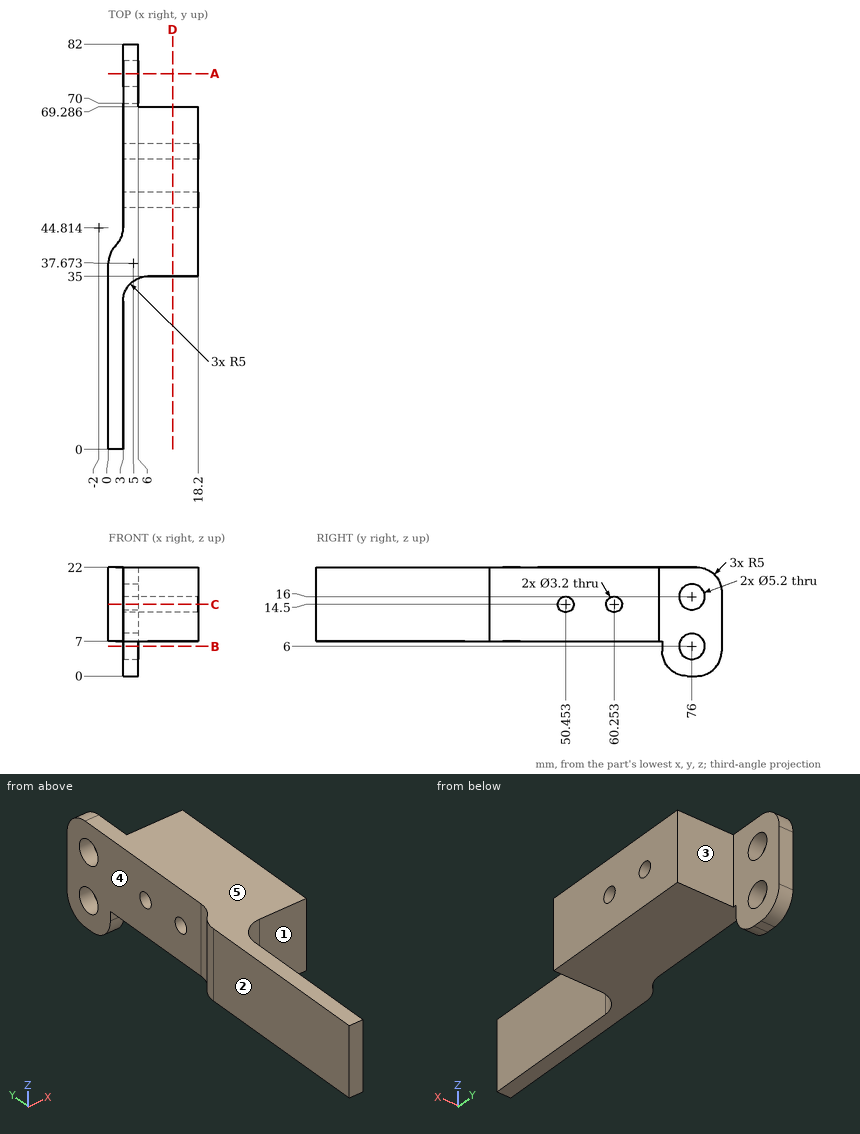
The drawing under review shows one solid part. Ordinate dimensions are in mm from its lowest x, y, z. A direction names the side the tool comes from. Give positions to 0.01 mm unless a question says otherwise; leave off trailing zeros. Loops run counter-clockwise (first coordinate to the right, second up) from the corner with the lowest first, then second, coordinate; pieces in that order, holes last. Notation, with made-up numbers: M 58,12.5 L 73,12.5 A35 cw 73,45.5 Z; hole C 55.25,-31.75 d1. An arc over 180 degrees is marked long. Return JSON: item names as keys, results as strings. Group by question number.
Item 1: We need section C-C (z = 14.5). Give the boundary of the cut face in (x, y).
Item 2: We need section A-A (y = 76). Give the boundary of the cut face in (x, z), and give its area (3 significant figures).
Item 3: We need section B-B (z = 6). Give the boundary of the cut face in (x, y), and give its area (3 significant figures).
Item 4: For probe 1 along Z at (x, y) = (13, 50.5); probe 2 along Y at (x, z) = (3.65, 6); probe 3 along Y at (x, z) = (11.75, 21.25), list the stretches that pass through material, from the lowest coordinate up.
Item 5: Insertion check: pin 1 Ø12 at (y, z) = (17, 11.5) entering from +X; pin 2 Ø6.5 at (y, z) = (77.5, 8) entering from +X; pin 3 Ø1.6 at (x, z) = (4.5, 6) entering from -Y. Each pin has a flat end and moves straight along its axis. Give the tip position at first contact, or say it passes through.
Item 6: Tool access review of the marked faces 1, 2, 3, 4 and 5: name each direction out of +Z, -Z, +X, -X, +Y, -Y from which nothing blocks a thin tool from reaching the whole face with its end or side.
Item 7: We need section D-D (x = 13). Give the boundary of the cut face in (y, z), and give its area (3 significant figures).
Output:
{
 "1": {"outline": "M 0,0 L 3,0 L 3,30 A5 cw 8,35 L 18.2,35 L 18.2,48.85 L 3,48.85 L 3,44.81 A5 cw 1.5,41.24 A5 ccw 0,37.67 Z; M 3,52.05 L 18.2,52.05 L 18.2,58.65 L 3,58.65 Z; M 3,61.85 L 18.2,61.85 L 18.2,69.29 L 6,69.29 L 6,73.88 L 3,73.88 Z; M 3,78.12 L 6,78.12 L 6,82 L 3,82 Z"},
 "2": {"outline": "M 3,0 L 6,0 L 6,3.4 L 3,3.4 Z; M 3,8.6 L 6,8.6 L 6,13.4 L 3,13.4 Z; M 3,18.6 L 6,18.6 L 6,22 L 3,22 Z", "area": "34.8 mm^2"},
 "3": {"outline": "M 3,70 L 6,70 L 6,73.4 L 3,73.4 Z; M 3,78.6 L 6,78.6 L 6,82 L 3,82 Z", "area": "20.4 mm^2"},
 "4": {"probe 1": "z = 7 to 12.9, 16.1 to 22", "probe 2": "y = 70 to 73.4, 78.6 to 82", "probe 3": "y = 35 to 69.29"},
 "5": {"pin 1": "stops at x = 3", "pin 2": "stops at x = 6", "pin 3": "stops at y = 70"},
 "6": {"face 1": "+Z, -Z, +X, -Y", "face 2": "+Z, -Z, -X, +Y, -Y", "face 3": "+Z, -Z, +X, +Y", "face 4": "+Z, -Z, -X, +Y", "face 5": "+Z, +X, -X, +Y, -Y"},
 "7": {"outline": "M 35,7 L 69.29,7 L 69.29,22 L 35,22 Z; hole C 50.45,14.5 d3.2; hole C 60.25,14.5 d3.2", "area": "498 mm^2"}
}
